from build123d import *

# Parameters (mm, degrees)
F2_DEPTH = 7


with BuildPart() as f2:
    # F1 (on Top) → F2 (new body)
    with BuildSketch(Plane.XY):
        with BuildLine():
            Line((0, 0), (-5, 0))
            Line((-5, 0), (-5, 5))
            Line((-5, 5), (-5, 8.660254))
            ThreePointArc((-5, 8.660254), (-8.660254, 5), (-10, 0))
            ThreePointArc((-10, 0), (-8.660254, -5), (-5, -8.660254))
            ThreePointArc((-5, -8.660254), (0, -10), (5, -8.660254))
            ThreePointArc((5, -8.660254), (8.660254, -5), (10, 0))
            ThreePointArc((10, 0), (8.660254, 5), (5, 8.660254))
            Line((5, 8.660254), (5, 5))
            Line((5, 5), (5, 0))
            Line((5, 0), (0, 0))
        make_face()
        with BuildLine():
            Line((24.150635, -8.169873), (10, 0))
            ThreePointArc((10, 0), (8.660254, -5), (5, -8.660254))
            Line((5, -8.660254), (19.150635, -16.830127))
            Line((19.150635, -16.830127), (24.150635, -8.169873))
        make_face()
        Polygon((5, 5), (0, 0), (5, 0), align=None)
        Polygon((-5, 5), (-5, 0), (0, 0), align=None)
        with BuildLine():
            Line((-5, 5), (0, 0))
            Line((0, 0), (5, 5))
            Line((5, 5), (5, 8.660254))
            ThreePointArc((5, 8.660254), (0, 10), (-5, 8.660254))
            Line((-5, 8.660254), (-5, 5))
        make_face()
        with BuildLine():
            Line((-5, 25), (-5, 8.660254))
            ThreePointArc((-5, 8.660254), (0, 10), (5, 8.660254))
            Line((5, 8.660254), (5, 25))
            Line((5, 25), (-5, 25))
        make_face()
        with BuildLine():
            ThreePointArc((-5, -8.660254), (-8.660254, -5), (-10, 0))
            Line((-10, 0), (-24.150635, -8.169873))
            Line((-24.150635, -8.169873), (-19.150635, -16.830127))
            Line((-19.150635, -16.830127), (-5, -8.660254))
        make_face()
    extrude(amount=F2_DEPTH)


solid = f2.part
Design review of the part built by this model. Coordinates are the model's own, in mm. A direction names the side the tool comes from. Round coordinates to 2 decimals unless told otherwise and drop trailing zeros. Loops run counter-clockwise (first coordinate to the right, second up) from the corner with the lowest first, then second, coordinate; pieces in that order, holes last. Notation, with made-up numbers: (89, 45) - (93, 45) arc R10 cw to (93, 59) - close; hole circle Ø8 at (33, -7.5). An arc over 180 degrees is marked (long way). One line per question, with ' | ' between items.
1. We need section A-A, the plane z = 3.25. State the section outline as (x, y) points, and give its area (3 significant figures).
Results are:
outline: (-24.15, -8.17) - (-19.15, -16.83) - (-5, -8.66) arc R10 ccw to (5, -8.66) - (19.15, -16.83) - (24.15, -8.17) - (10, 0) arc R10 ccw to (5, 8.66) - (5, 25) - (-5, 25) - (-5, 8.66) arc R10 ccw to (-10, 0) - close | area: 777 mm²
2. Clearance check with flat-ended pins moving along their axes: P1, Ø2, axis at y = 13, z = 3, coming from the -X side; P2, Ø1, axis at x = 7.5, z = 3.5, coming from the -Y side; P3, Ø2, axis at x = 11, z = 1, coming from the -Y side. State where each tip first meets the part, or that it passes through.
Results are:
P1: stops at x = -5 | P2: stops at y = -10.39 | P3: stops at y = -12.7
3. We need section B-B, the plane y = 14. State the section outline as (x, z) points, and give its area (3 significant figures).
Results are:
outline: (-5, 0) - (5, 0) - (5, 7) - (-5, 7) - close | area: 70.0 mm²
4. We need section C-C, the plane x = -14.5. State the section outline as (y, z) points.
Results are:
outline: (-14.15, 0) - (-2.6, 0) - (-2.6, 7) - (-14.15, 7) - close
5. For L1, parallel to Y at x = 0, z = 1.5; L2, parallel to X at y = 19.5, z = 2.5; L3, parallel to X at y = -12.5, z = 4.25, list the stretches that pass through material, from the lowest coordinate up. Write a range as [from, to].
Results are:
L1: y = [-10, 25] | L2: x = [-5, 5] | L3: x = [-21.65, -11.65], [11.65, 21.65]
6. Draft analysis for pull direction X (two halves, no side actions). For faces 1 (the face through (21.616, -12.561, 3.451)), 2 (the face through (0, 0, 0)), 3 (the face through (-8.6, 5.1, 3.5)), 4 (the face through (0, -10, 3)), state which applies: released by +X, released by -X, zero draft, split by the parting line, or undercut.
Results are:
face 1: released by +X | face 2: zero draft | face 3: released by -X | face 4: undercut
7. For faces 5 (the face through (-21.686, -12.439, 3.451)), 6 (the face through (-5, 17, 3)), 7 (the face through (12, -12.7, 3.5)), 8 (the face through (0, 25, 3)), 9 (the face through (5, 17, 3)), list the 3-axis set-ups (+Z, -Z, +X, -X, +Y, -Y) from which the entire face can be reached by the end or side of a thin tool; tool diameter is ignored.
Results are:
face 5: +Z, -Z, -X, -Y | face 6: +Z, -Z, -X, +Y | face 7: +Z, -Z, -Y | face 8: +Z, -Z, +X, -X, +Y | face 9: +Z, -Z, +X, +Y
